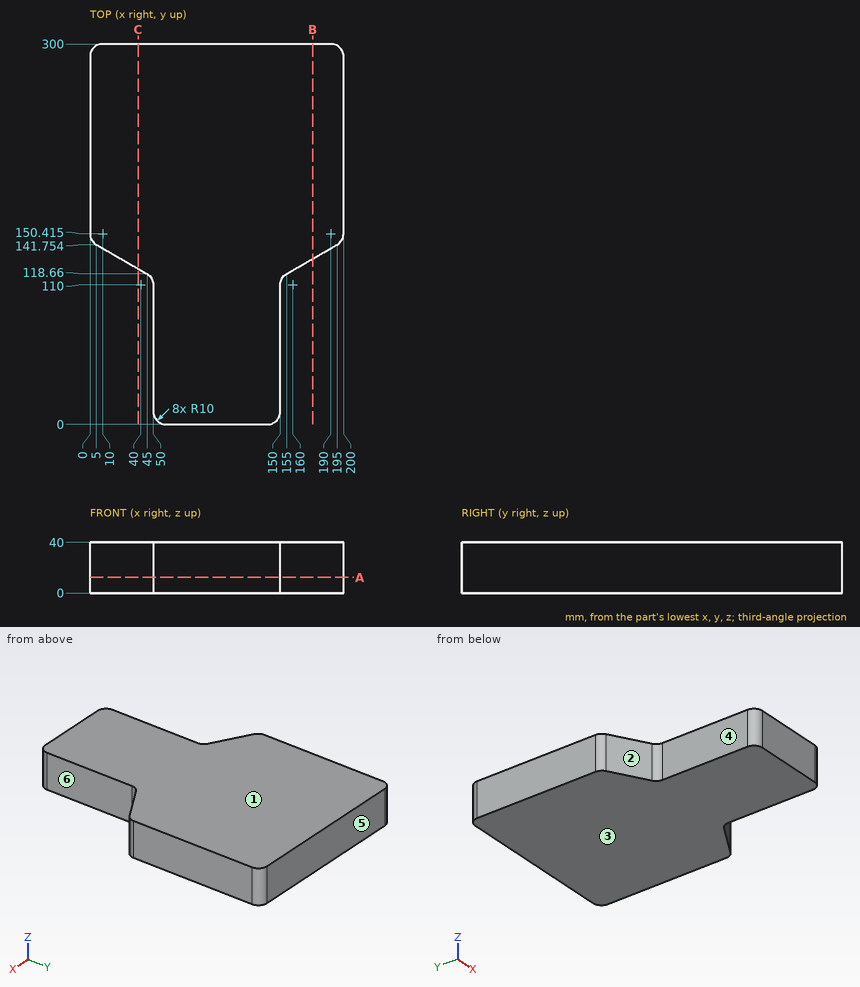
Can you work these out from the drawing? Everything is in mm from the part's minimum corner. A direction names the side the tool comes from. Coordinates: 2 decimals unless noted, no trailing zeros. Loops run counter-clockwise (first coordinate to the right, second up) from the corner with the lowest first, then second, coordinate; pieces in that order, holes last. Notation, with made-up numbers: M 30,-15 L 34,-15 A14 cw 34,5 Z; hole C 29,19 d9. An arc over 180 degrees is marked long. One line per item, written item: value.
1. Thinking about a two-plate mould opening in Z: for the marked faces 1, 2 and 3, which applies, +Z half, -Z half, draft (parallel to the pull), parting line (faces both ways), or undercut?
Geometry says:
face 1: +Z half
face 2: draft
face 3: -Z half
2. Please list where these lines run through material, in increasing order: probe 1 along X at (y, z) = (87.5, 21); probe 2 along Y at (x, z) = (163, 30); probe 3 along X at (y, z) = (133, 20) (1 decimal).
Geometry says:
probe 1: x = 50 to 150
probe 2: y = 123.28 to 300
probe 3: x = 20.2 to 179.8
3. Imagine slicing it at C-C (x = 38). List the corners of the cut face in (y, z) for me.
Geometry says:
outline: M 122.7,0 L 300,0 L 300,40 L 122.7,40 Z
4. Imagine slicing it at B-B (x = 175.5). List the corners of the cut face in (y, z) for me (1 decimal).
Geometry says:
outline: M 130.5,0 L 300,0 L 300,40 L 130.5,40 Z
5. On a 3-axis mill with a long thin cutter (end or side, diameter ignored), from which of +Z, -Z, +X, -X, +Y, -Y can I reach the whole of each face in a straight line? I mean the marked faces 4, 5 and 6. Say none if no direction works.
Geometry says:
face 4: +Z, -Z, -X, -Y
face 5: +Z, -Z, +X, -X, +Y
face 6: +Z, -Z, +X, -Y
6. Will these pins go through, and if not, where does the flat tip stop? pin 1 Ø1.5 at (y, z) = (36, 20) entering from -X; pin 2 Ø5 at (y, z) = (36.5, 35) entering from +X.
Geometry says:
pin 1: stops at x = 50
pin 2: stops at x = 150
7. Imagine slicing it at A-A (z = 12.5). List the corners of the cut face in (x, y) for me (1 decimal), and give its area (3 significant figures).
Geometry says:
outline: M 0,150.4 A10 ccw 5,141.8 L 45,118.7 A10 cw 50,110 L 50,10 A10 ccw 60,0 L 140,0 A10 ccw 150,10 L 150,110 A10 cw 155,118.7 L 195,141.8 A10 ccw 200,150.4 L 200,290 A10 ccw 190,300 L 10,300 A10 ccw 0,290 Z
area: 46,900 mm2
